Geometry: final body of the model. Coordinates: model frame, mm. A direction names the side the tool comes from. Round coordinates to 2 decimals unless told otherwise and drop trailing zeros. Loops run counter-clockwise (first coordinate to the right, second up) from the corner with the lowest first, then second, coordinate; pieces in that order, holes last. Notation, with made-up numbers: (74, 30.5) - (100, 30.5) arc R30 cw to (100, 67.5) - close; hole circle Ø9 at (83.25, 51.25). An arc over 180 degrees is marked (long way). Answer as a JSON object with one key per item and string values. Group by question number.
Item 1: Section C-C (y = 20). Return the cut outline in (x, z).
Item 2: Reachability of faces 1 (the face through (27, 40, 49)), 2 (the face through (47.5, 20, 83)), 3 (the face through (42.5, 24.2, 27.2)) from +Z, -Z, +X, -X, +Y, -Y: full face, straight path, thin tool, end or side. Return the list, or none.
Item 3: Line query: line 1 (Z direction, x = 4, y = 20); line 2 (X direction, y = 8.5, z = 23); line 3 (X direction, y = 33.5, z = 75). Output: solid intervals per line, ascending.
Item 4: Section A-A (z = 30.5). Return the cut outline in (x, y), plus the area to 3 significant figures.
Item 5: Section B-B (z = 90). Return the cut outline in (x, y).
Item 6: Section D-D (y = 33). Return the cut outline in (x, z), plus the area to 3 significant figures.
Item 7: Draft query along Y for faces 4 (the face through (3.803, 19.133, 86.095)), 5 (the face through (28, 20, 45)), 6 (the face through (27, 0, 49)). Return one class per face: released by +Y, released by -Y, zero draft, split by the parting line, or undercut.
Item 8: First-contact query: pin 1 (1.5 mm diameter, centred on x = 26, y = 21.5, fed in from -Z). Flat tip, straight axial feed; report the tip coordinate or a pass-through.
```python
from build123d import *

# Parameters (mm, degrees)
SKETCH1_W           = 55
SKETCH1_H           = 40
BOSS_EXTRUDE1_DEPTH = 100
SKETCH2_W           = 40
SKETCH2_H           = 40
CUT_EXTRUDE1_DEPTH  = 35
SKETCH3_R           = 4
SKETCH3_R_2         = 8
CUT_EXTRUDE2_DEPTH  = 121.933866224
SKETCH4_W           = 30
SKETCH4_H           = 40
CUT_EXTRUDE3_DEPTH  = 45


with BuildPart() as part:
    # Sketch1 → Boss-Extrude1 (new body)
    with BuildSketch(Plane.XY):
        with Locations((27.5, 20)):
            Rectangle(SKETCH1_W, SKETCH1_H)
    extrude(amount=BOSS_EXTRUDE1_DEPTH)

    # Sketch2 → Cut-Extrude1 (cut)
    with BuildSketch(Plane.XY.offset(100)):
        with Locations((27.5, 20)):
            Rectangle(SKETCH2_W, SKETCH2_H)
    extrude(amount=-CUT_EXTRUDE1_DEPTH, mode=Mode.SUBTRACT)

    # Sketch3 → Cut-Extrude2 (cut, through all)
    with BuildSketch(Plane(origin=(55, 0, 0), x_dir=(0, 0, -1), z_dir=(1, 0, 0))):
        with Locations(Location((-90, 20, 0), (0, 0, 90))):
            Circle(SKETCH3_R)
        with Locations(Location((-20, 20, 0), (0, 0, 90))):
            Circle(SKETCH3_R_2)
    extrude(amount=-CUT_EXTRUDE2_DEPTH, mode=Mode.SUBTRACT)

    # Sketch4 → Cut-Extrude3 (cut)
    with BuildSketch(Plane(origin=(0, 0, 0), x_dir=(-1, 0, 0), z_dir=(0, 0, -1))):
        with Locations((-27.5, 20)):
            Rectangle(SKETCH4_W, SKETCH4_H)
    extrude(amount=-CUT_EXTRUDE3_DEPTH, mode=Mode.SUBTRACT)


solid = part.part
```
Values:
{
 "1": {"outline": "(0, 0) - (12.5, 0) - (12.5, 12) - (0, 12) - close; (0, 28) - (12.5, 28) - (12.5, 45) - (42.5, 45) - (42.5, 28) - (55, 28) - (55, 86) - (47.5, 86) - (47.5, 65) - (7.5, 65) - (7.5, 86) - (0, 86) - close; (0, 94) - (7.5, 94) - (7.5, 100) - (0, 100) - close; (42.5, 0) - (55, 0) - (55, 12) - (42.5, 12) - close; (47.5, 94) - (55, 94) - (55, 100) - (47.5, 100) - close"},
 "2": {"face 1": "+Z, -Z, +X, -X, +Y", "face 2": "+Z, +Y, -Y", "face 3": "-Z, +Y, -Y"},
 "3": {"line 1": "z = 0 to 12, 28 to 86, 94 to 100", "line 2": "x = 0 to 12.5, 42.5 to 55", "line 3": "x = 0 to 7.5, 47.5 to 55"},
 "4": {"outline": "(0, 0) - (12.5, 0) - (12.5, 40) - (0, 40) - close; (42.5, 0) - (55, 0) - (55, 40) - (42.5, 40) - close", "area": "1,000 mm^2"},
 "5": {"outline": "(0, 0) - (7.5, 0) - (7.5, 16) - (0, 16) - close; (0, 24) - (7.5, 24) - (7.5, 40) - (0, 40) - close; (47.5, 0) - (55, 0) - (55, 16) - (47.5, 16) - close; (47.5, 24) - (55, 24) - (55, 40) - (47.5, 40) - close"},
 "6": {"outline": "(0, 0) - (12.5, 0) - (12.5, 45) - (42.5, 45) - (42.5, 0) - (55, 0) - (55, 100) - (47.5, 100) - (47.5, 65) - (7.5, 65) - (7.5, 100) - (0, 100) - close", "area": "2,750 mm^2"},
 "7": {"face 4": "undercut", "face 5": "zero draft", "face 6": "released by -Y"},
 "8": {"pin 1": "stops at z = 45"}
}
